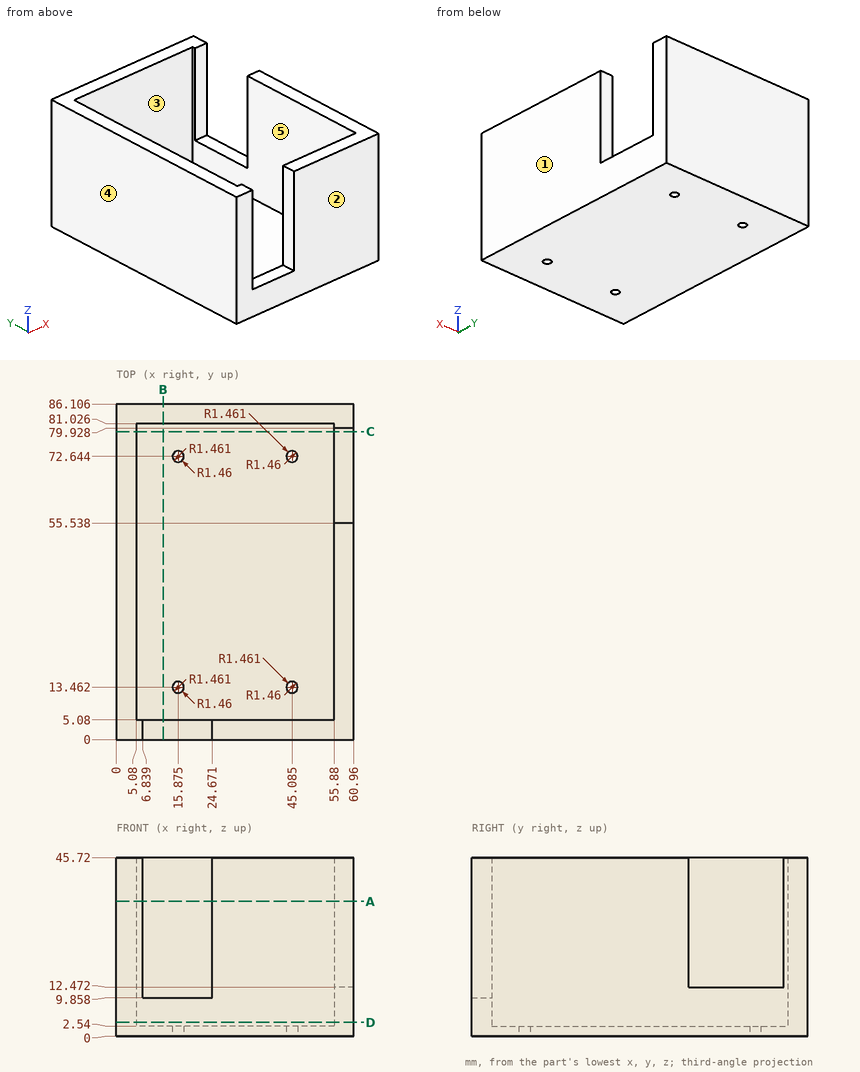
Check sheet for the drawn part. Datum: minimum x, y, z corner. Units: mm. A direction names the side the tool comes from. Give positions to 0.01 mm unless a question says otherwise; leave off trailing zeros. Order: outer loops, then holes, each group sorted by start corner. A loop starts at its lowest first (then second) coordinate and runs counter-clockwise, first axis right, second up. Notation, with made-up numbers: (-40, 11) -> (-32, 11) arc R7 cw to (-32, 15) -> close; hole circle Ø4 at (22.25, 1.5). An arc over 180 degrees is marked (long way). Use a Markdown table: item, result.
1) Section check D-D, the plane z = 3.5. Record the boundary of the cut face in (x, y) (1 decimal).
Results:
| item | result |
|---|---|
| outline | (0, 0) -> (61, 0) -> (61, 86.1) -> (0, 86.1) -> close; hole (5.1, 5.1) -> (55.9, 5.1) -> (55.9, 81) -> (5.1, 81) -> close |
2) Tool access check on the marked faces 4 and 5. Record the directions out of +Z, -Z, +X, -X, +Y, -Y that give a thin tool (end or side, any length) a straight path to the whole face; none if there is none.
Results:
| item | result |
|---|---|
| face 4 | +Z, -Z, -X, +Y, -Y |
| face 5 | +Z |
3) Section check B-B, the plane x = 12. Record the boundary of the cut face in (y, z) (1 decimal).
Results:
| item | result |
|---|---|
| outline | (0, 0) -> (86.1, 0) -> (86.1, 45.7) -> (81, 45.7) -> (81, 2.5) -> (5.1, 2.5) -> (5.1, 9.9) -> (0, 9.9) -> close |
4) Mould release check, pull along Y, two halves, no side actions. Record for the marked faces 1, 2 and 3: pulls with the +Y half, pulls with the -Y half, needs draft (parallel to the pull), parting line crosses it, or undercut.
Results:
| item | result |
|---|---|
| face 1 | needs draft |
| face 2 | pulls with the -Y half |
| face 3 | undercut |
5) Material ranges on probe 1 along X at (y, z) = (74, 9); probe 2 along Y at (x, z) = (5.5, 17.5) (1 decimal); probe 3 along Z at (x, y) = (35, 72), recorded low to high.
Results:
| item | result |
|---|---|
| probe 1 | 0 to 5.08, 55.88 to 60.96 |
| probe 2 | 0 to 5.1, 81 to 86.1 |
| probe 3 | 0 to 2.54 |
6) Depth check by flat-ended pin: pin 1 Ø1.5 at (x, y) = (14, 2) entering from +Z; pin 2 Ø1.5 at (x, y) = (27, 64.5) entering from +Z; pin 3 Ø2.5 at (x, y) = (57.5, 70.5) entering from +Z. Enter the tip coordinate at first touch or a pass-through.
Results:
| item | result |
|---|---|
| pin 1 | z = 9.86 |
| pin 2 | z = 2.54 |
| pin 3 | z = 12.47 |
7) Section check A-A, the plane z = 34.5. Record the boundary of the cut face in (x, y) (1 decimal).
Results:
| item | result |
|---|---|
| outline | (0, 0) -> (6.8, 0) -> (6.8, 5.1) -> (5.1, 5.1) -> (5.1, 81) -> (55.9, 81) -> (55.9, 79.9) -> (61, 79.9) -> (61, 86.1) -> (0, 86.1) -> close; (24.7, 0) -> (61, 0) -> (61, 55.5) -> (55.9, 55.5) -> (55.9, 5.1) -> (24.7, 5.1) -> close |
8) Section check C-C, the plane y = 79. Record the boundary of the cut face in (x, z).
Results:
| item | result |
|---|---|
| outline | (0, 0) -> (60.96, 0) -> (60.96, 12.47) -> (55.88, 12.47) -> (55.88, 2.54) -> (5.08, 2.54) -> (5.08, 45.72) -> (0, 45.72) -> close |
